CAD build for the part. Positions are in the model's coordinates, mm. A direction names the side the tool comes from. Give positions to 0.01 mm unless a question says otherwise; leave off trailing zeros. Loops run counter-clockwise (first coordinate to the right, second up) from the corner with the lowest first, then second, coordinate; pieces in that order, holes last. Notation, with made-up numbers: M -3.5,-27.5 L 11.5,-27.5 A24 ccw 11.5,-15.5 Z; hole C -22,15.25 d8. An arc over 180 degrees is marked long. Answer as CSV lines item,"result".
from build123d import *

# Parameters (mm, degrees)
SKETCH1_W           = 40
SKETCH1_H           = 11.5
BOSS_EXTRUDE1_DEPTH = 1
CUT_EXTRUDE1_DEPTH  = 1
FILLET1_R           = 2
FILLET2_R           = 4
FILLET3_R           = 2
CUT_EXTRUDE2_DEPTH  = 1
CUT_EXTRUDE3_DEPTH  = 1
FILLET4_R           = 2
FILLET5_R           = 7
FILLET6_R           = 4
FILLET7_R           = 4
SKETCH5_R           = 1.5
SKETCH5_R_2         = 1.501453264
CUT_EXTRUDE4_DEPTH  = 1


with BuildPart() as part:
    # Sketch1 → Boss-Extrude1 (new body)
    with BuildSketch(Plane(origin=(0, 0, 0), x_dir=(1, 0, 0), z_dir=(0, 1, 0))):
        Rectangle(SKETCH1_W, SKETCH1_H)
    extrude(amount=BOSS_EXTRUDE1_DEPTH)

    # Sketch2 → Cut-Extrude1 (cut)
    with BuildSketch(Plane(origin=(0, 1, 0), x_dir=(1, 0, 0), z_dir=(0, 1, 0))):
        Polygon((-20, 4.177870703), (0, 5.75), (-20, 5.75), align=None)
        Polygon((20, 5.75), (0, 5.75), (20, 4.177870703), align=None)
    extrude(amount=-CUT_EXTRUDE1_DEPTH, mode=Mode.SUBTRACT)

    # Fillet1
    fillet1_edges = [part.edges().sort_by_distance(p)[0] for p in [
        (0, 0.5, -5.75),
    ]]
    fillet(fillet1_edges, radius=FILLET1_R)

    # Fillet2
    fillet2_edges = [part.edges().sort_by_distance(p)[0] for p in [
        (20, 0.5, -4.177870703),
    ]]
    fillet(fillet2_edges, radius=FILLET2_R)

    # Fillet3
    fillet3_edges = [part.edges().sort_by_distance(p)[0] for p in [
        (-20, 0.5, -4.177870703),
    ]]
    fillet(fillet3_edges, radius=FILLET3_R)

    # Sketch3 → Cut-Extrude2 (cut)
    with BuildSketch(Plane(origin=(0, 1, 0), x_dir=(1, 0, 0), z_dir=(0, 1, 0))):
        Polygon((-20, 2.328914172), (-19.016050198, -5.75), (-20, -5.75), align=None)
    extrude(amount=-CUT_EXTRUDE2_DEPTH, mode=Mode.SUBTRACT)

    # Sketch4 → Cut-Extrude3 (cut)
    with BuildSketch(Plane(origin=(0, 1, 0), x_dir=(1, 0, 0), z_dir=(0, 1, 0))):
        Polygon((4.487841755, -0.29957878), (-19.016050198, -5.75), (10.444676757, -5.75), align=None)
        Polygon((20, -3.02478939), (10.444676757, -5.75), (20, -5.75), align=None)
    extrude(amount=-CUT_EXTRUDE3_DEPTH, mode=Mode.SUBTRACT)

    # Fillet4
    fillet4_edges = [part.edges().sort_by_distance(p)[0] for p in [
        (-19.016050198, 0.5, 5.75),
    ]]
    fillet(fillet4_edges, radius=FILLET4_R)

    # Fillet5
    fillet5_edges = [part.edges().sort_by_distance(p)[0] for p in [
        (4.487841755, 0.5, 0.29957878),
    ]]
    fillet(fillet5_edges, radius=FILLET5_R)

    # Fillet6
    fillet6_edges = [part.edges().sort_by_distance(p)[0] for p in [
        (10.444676757, 0.5, 5.75),
    ]]
    fillet(fillet6_edges, radius=FILLET6_R)

    # Fillet7
    fillet7_edges = [part.edges().sort_by_distance(p)[0] for p in [
        (20, 0.5, 3.02478939),
    ]]
    fillet(fillet7_edges, radius=FILLET7_R)

    # Sketch5 → Cut-Extrude4 (cut)
    with BuildSketch(Plane(origin=(0, 1, 0), x_dir=(1, 0, 0), z_dir=(0, 1, 0))):
        with Locations(Location((-17.048407867, 1.6240543, 0), (0, 0, 270))):
            Circle(SKETCH5_R)
        with Locations(Location((16.951592133, 1.6240543, 0), (0, 0, 270))):
            Circle(SKETCH5_R_2)
    extrude(amount=-CUT_EXTRUDE4_DEPTH, mode=Mode.SUBTRACT)


solid = part.part
1) Band-saw the part on A-A on y = 0.8. Give the cut face in (x, z).
Answer below:
outline,"M -20,-2.33 A2 ccw -18.16,-4.32 L -0.16,-5.74 A2 ccw 0.16,-5.74 L 16.31,-4.47 A4 ccw 20,-0.48 L 20,0.01 A4 ccw 17.1,3.85 L 12.59,5.14 A4 ccw 8.8,4.24 L 7.21,2.79 A7 cw 0.9,1.13 L -16.85,5.25 A2 ccw -19.29,3.54 Z; hole C -17.05,-1.62 d3; hole C 16.95,-1.62 d3"
2) Mould opens along X. For faces 1 (the face through (0, 1, 0)), 2 (the face through (18.909, 0.493, -3.226)), 3 (the face through (-15.78, 0.51, -0.82)), 4 (the face through (4.211, 0.493, 1.168)) say: +X half, -X half, draft (parallel to the pull), parting line (faces both ways), or undercut.
Answer below:
face 1,"draft"
face 2,"+X half"
face 3,"undercut"
face 4,"undercut"
3) Drill centre lines: line 1 (X direction, y = 0.3, z = -2.75); line 2 (X direction, y = 0.4, z = -0.5); line 3 (Z direction, x = -16, y = 0.95). Where is each one in solid material? Low to high. Write a range as from..to.
Answer below:
line 1,"x = -19.96..-18.04, -16.06..15.96, 17.94..19.29"
line 2,"x = -19.78..-18.04, -16.06..15.96, 17.95..20"
line 3,"z = -4.49..-2.7, -0.55..5.05"
4) Band-saw the part on D-D on x = 3.5. Give the cut face in (y, z), and give its area (3 significant figures).
Answer below:
outline,"M 0,-5.47 L 1,-5.47 L 1,1.03 L 0,1.03 Z"
area,"6.50 mm^2"
5) Band-saw the part on B-B on z = 4.75. Give the cut face in (x, y).
Answer below:
outline,"M -18.68,0 L -14.7,0 L -14.7,1 L -18.68,1 Z; M 9.49,0 L 13.95,0 L 13.95,1 L 9.49,1 Z"
6) Which spindle directions (+Z, -Z, +X, -X, +Y, -Y) get a long thin tool onto all of the face, cutting with end or side? Do faces 5 (the face through (-7.85, 0.51, 3.16)), 6 (the face through (0, 0, 0)). Say none if no direction does.
Answer below:
face 5,"+Z, +Y, -Y"
face 6,"+Z, -Z, +X, -X, -Y"
7) Band-saw the part on C-C on x = -9. Give the cut face in (y, z).
Answer below:
outline,"M 0,-5.04 L 1,-5.04 L 1,3.43 L 0,3.43 Z"
